```python
from build123d import *

# Parameters (mm, degrees)
F3_DEPTH = 6.35
F1_DEPTH = 2.54


with BuildPart() as f3:
    # F2 (on face) → F3 (new body)
    with BuildSketch(Plane.XY):
        with BuildLine():
            ThreePointArc((44.544026, 36.572959), (42.684154, 41.063087), (38.194026, 42.922959))
            Line((38.194026, 42.922959), (-39.380025, 42.922959))
            ThreePointArc((-39.380025, 42.922959), (-43.870153, 41.063087), (-45.730025, 36.572959))
            Line((-45.730025, 36.572959), (-45.730025, -13.405945))
            ThreePointArc((-45.730025, -13.405945), (-43.870153, -17.896073), (-39.380025, -19.755945))
            Line((-39.380025, -19.755945), (38.194026, -19.755945))
            ThreePointArc((38.194026, -19.755945), (42.684154, -17.896073), (44.544026, -13.405945))
            Line((44.544026, -13.405945), (44.544026, 36.572959))
        make_face()
        with BuildLine():
            ThreePointArc((-43.190025, 36.572959), (-42.074101, 39.267036), (-39.380025, 40.382959))
            Line((-39.380025, 40.382959), (38.194026, 40.382959))
            ThreePointArc((38.194026, 40.382959), (40.888103, 39.267036), (42.004026, 36.572959))
            Line((42.004026, 36.572959), (42.004026, -13.405945))
            ThreePointArc((42.004026, -13.405945), (40.888103, -16.100021), (38.194026, -17.215945))
            Line((38.194026, -17.215945), (-39.380025, -17.215945))
            ThreePointArc((-39.380025, -17.215945), (-42.074101, -16.100021), (-43.190025, -13.405945))
            Line((-43.190025, -13.405945), (-43.190025, 36.572959))
        make_face(mode=Mode.SUBTRACT)
    extrude(amount=F3_DEPTH)

    # F0 (on Top) → F1 (join)
    with BuildSketch(Plane.XY):
        with BuildLine():
            Line((38.194026, 42.922959), (-39.380025, 42.922959))
            ThreePointArc((-39.380025, 42.922959), (-43.870153, 41.063087), (-45.730025, 36.572959))
            Line((-45.730025, 36.572959), (-45.730025, -13.405945))
            ThreePointArc((-45.730025, -13.405945), (-43.870153, -17.896073), (-39.380025, -19.755945))
            Line((-39.380025, -19.755945), (38.194026, -19.755945))
            ThreePointArc((38.194026, -19.755945), (42.684154, -17.896073), (44.544026, -13.405945))
            Line((44.544026, -13.405945), (44.544026, 36.572959))
            ThreePointArc((44.544026, 36.572959), (42.684154, 41.063087), (38.194026, 42.922959))
        make_face()
    extrude(amount=F1_DEPTH)


solid = f3.part
```
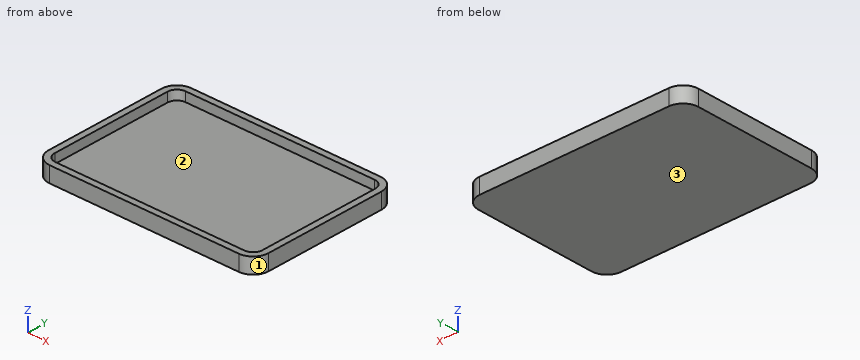
Design review of the part built by this model. Coordinates are the model's own, in mm. Face numbers are marked on the shaded views. Give positions to 0.01 mm unless a question says otherwise; leave off trailing zeros. Write each loop counter-clockwise with the first axis right and the second up, starting at its lowest first coordinate (ties: lowest second). Pieces come first, ordered by that corner, then holes. Notation, with made-up numbers: (-18.5, 37) - (31.5, 37) arc R10 cw to (31.5, 45) - close; hole circle Ø10 at (73.25, 87). An arc over 180 degrees is marked (long way). Return JSON: item names as keys, results as strings. Group by question number.
(1) Mouldability with a two-part tool opening along X and no side actions: class the marked faces 1, 2 and 3 as +X half, -X half, draft (parallel to the pull), parting line (faces both ways), or undercut.
(2) We need section A-A, the plane z = 3.5. Give the boundary of the cut face in (x, y), then the cut area to 3 significant figures.
(3) We need section B-B, the plane y = 31. Give the boundary of the cut face in (x, z), then the cut area to 3 significant figures.
(4) To check wall thickness, follow probe 1 along Y at (x, z) = (24, 5.75); probe 2 along X at (y, z) = (12, 6); probe 3 along Z at (x, y) = (22, -8). State the ranges of each line that lie inside material, in increasing order.
(5) We need section C-C, the plane x = -15. Give the boundary of the cut face in (y, z).
(6) Insertion check: pin 1 (12 mm diameter, centred on x = 13, y = 22.5, fed in from +Z). The pin has a flat end and moves straight along its axis. Give the tip position at first contact, or say it passes through.
Reported:
{
 "1": {"face 1": "+X half", "face 2": "undercut", "face 3": "draft"},
 "2": {"outline": "(-45.73, -13.41) arc R6.35 ccw to (-39.38, -19.76) - (38.19, -19.76) arc R6.35 ccw to (44.54, -13.41) - (44.54, 36.57) arc R6.35 ccw to (38.19, 42.92) - (-39.38, 42.92) arc R6.35 ccw to (-45.73, 36.57) - close; hole (-43.19, -13.41) arc R3.81 ccw to (-39.38, -17.22) - (38.19, -17.22) arc R3.81 ccw to (42, -13.41) - (42, 36.57) arc R3.81 ccw to (38.19, 40.38) - (-39.38, 40.38) arc R3.81 ccw to (-43.19, 36.57) - close", "area": "729 mm2"},
 "3": {"outline": "(-45.73, 0) - (44.54, 0) - (44.54, 6.35) - (42, 6.35) - (42, 2.54) - (-43.19, 2.54) - (-43.19, 6.35) - (-45.73, 6.35) - close", "area": "249 mm2"},
 "4": {"probe 1": "y = -19.76 to -17.22, 40.38 to 42.92", "probe 2": "x = -45.73 to -43.19, 42 to 44.54", "probe 3": "z = 0 to 2.54"},
 "5": {"outline": "(-19.76, 0) - (42.92, 0) - (42.92, 6.35) - (40.38, 6.35) - (40.38, 2.54) - (-17.22, 2.54) - (-17.22, 6.35) - (-19.76, 6.35) - close"},
 "6": {"pin 1": "stops at z = 2.54"}
}
